```python
from build123d import *

# Parameters (mm, degrees)
F1_DEPTH = 63.5
F0_W     = 25.4
F0_H     = 19.05
F2_DEPTH = 25.4
F3_DEPTH = 7.9375


with BuildPart() as f1:
    # F0 (on Front) → F1 (new body, symmetric)
    with BuildSketch(Plane.XZ):
        Polygon((-41.275, 9.525), (-41.275, -9.525), (41.275, -9.525), (41.275, 9.525), (22.225, 9.525), align=None)
    extrude(amount=F1_DEPTH, both=True)

    # F0 (on Front) → F2 (join, symmetric)
    with BuildSketch(Plane.XZ):
        with BuildLine():
            Line((22.225, 9.525), (41.275, 9.525))
            Line((41.275, 9.525), (41.275, 27.0002))
            ThreePointArc((41.275, 27.0002), (45.9246798487, 38.2255201513), (57.15, 42.8752))
            Line((57.15, 42.8752), (60.325, 42.8752))
            Line((60.325, 42.8752), (60.325, 61.9252))
            Line((60.325, 61.9252), (57.15, 61.9252))
            add(Edge.make_bspline(
                [(54.9287877913, 61.8544944459), (55.6719665289, 61.8841036278), (56.4124732559, 61.9076963905), (57.15, 61.9252)],
                knots=[109.6288950018, 109.6288950018, 109.6288950018, 109.6288950018, 111.5045361635, 111.5045361635, 111.5045361635, 111.5045361635], degree=3))
            ThreePointArc((54.9287877913, 61.8544944459), (31.6810830483, 50.8976871965), (22.225, 27.0002))
            Line((22.225, 27.0002), (22.225, 9.525))
        make_face()
        with Locations((73.025, 52.4002)):
            Rectangle(F0_W, F0_H)
        Polygon((85.725, 66.675), (85.725, 61.9252), (85.725, 42.8752), (85.725, 38.1), (111.125, 38.1), (111.125, 66.675), align=None)
    extrude(amount=F2_DEPTH, both=True)

    # F0 (on Front) → F3 (join, symmetric)
    with BuildSketch(Plane.XZ):
        with BuildLine():
            add(Edge.make_bspline(
                [(-41.275, 9.525), (-41.075235058, 37.8396194046), (11.490914143, 60.123874562), (54.9287877913, 61.8544944459)],
                knots=[0, 0, 0, 0, 109.6288950018, 109.6288950018, 109.6288950018, 109.6288950018], degree=3))
            Line((-41.275, 9.525), (22.225, 9.525))
            Line((22.225, 9.525), (22.225, 27.0002))
            ThreePointArc((22.225, 27.0002), (31.6810830483, 50.8976871965), (54.9287877913, 61.8544944459))
        make_face()
    extrude(amount=F3_DEPTH, both=True)


solid = f1.part
```
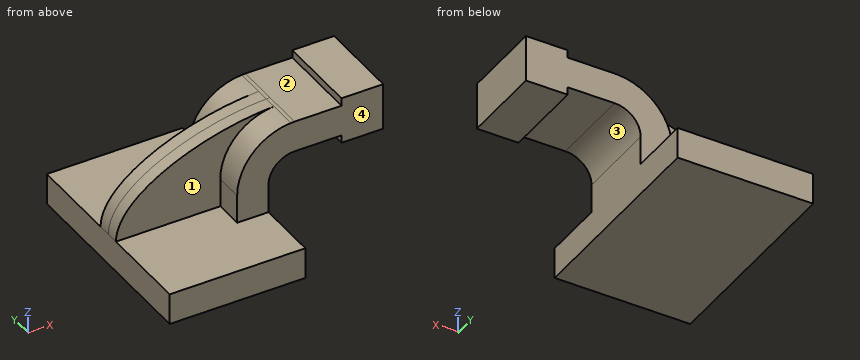
Could you check a few things on this model? Use its own coordinates, in mm. Face numbers are marked on the shaded views. A direction names the side the tool comes from. Coordinates: 2 decimals unless noted, no trailing zeros. Order: outer loops, then holes, each group sorted by start corner. A loop starts at its lowest first (then second) coordinate and runs counter-clockwise, first axis right, second up. Notation, with made-up numbers: M 12,14.5 L 19,14.5 A17 cw 19,45.5 Z; hole C 42.5,46.25 d11. An arc over 180 degrees is marked long. Use a Markdown table: item, result. Add a question column.
Q1. Which directions (+Z, -Z, +X, -X, +Y, -Y) give clear straight access to the entire face, cutting with the end or side of a thin tool? Please do the marked faces 1, 2, 3 and 4.
Q2. I'm going to push flat-ended pins straight in: pin 1 (18.5 mm diameter, centred on y = -3, z = -0.5, fed in from +X) (3 decimals); pin 2 (5 mm diameter, centred on x = 71, y = 26.5, fed in from +Z); pin 3 (20.5 mm diameter, centred on x = 103.5, y = -1, fed in from -Z). Where does each tip first touch, or does it pass through?
Q3. I want a section at A-A on x = 94.5. List the corners of the cut face in (y, z) for me (3 decimals), then the cut area to 3 significant figures.
Q4. I want a section at B-B on z = 4. List the corners of the cut face in (x, y) for me (3 decimals).
Q5. If I drill on L1, parallel to Z at x = 88, y = -23.5 (3 decimals); L2, parallel to X at y = 48.5, z = -2 (3 decimals); L3, parallel to X at y = -1.5, z = 63 (3 decimals), over which ranges is the centre line in solid material (lowest first)?
Checked values:
| question | item | result |
|---|---|---|
| 1 | face 1 | +Z, -X, -Y |
| 1 | face 2 | +Z, -X, +Y, -Y |
| 1 | face 3 | -Z, +Y, -Y |
| 1 | face 4 | +Z, +X, -X, -Y |
| 2 | pin 1 | x = 41.275 |
| 2 | pin 2 | z = 61.93 |
| 2 | pin 3 | z = 38.1 |
| 3 | outline | M -25.4,38.1 L 25.4,38.1 L 25.4,66.675 L -25.4,66.675 Z |
| 3 | area | 1,450 mm² |
| 4 | outline | M -41.275,-63.5 L 41.275,-63.5 L 41.275,63.5 L -41.275,63.5 Z |
| 5 | L1 | 38.1 to 66.675 |
| 5 | L2 | -41.275 to 41.275 |
| 5 | L3 | 85.725 to 111.125 |
